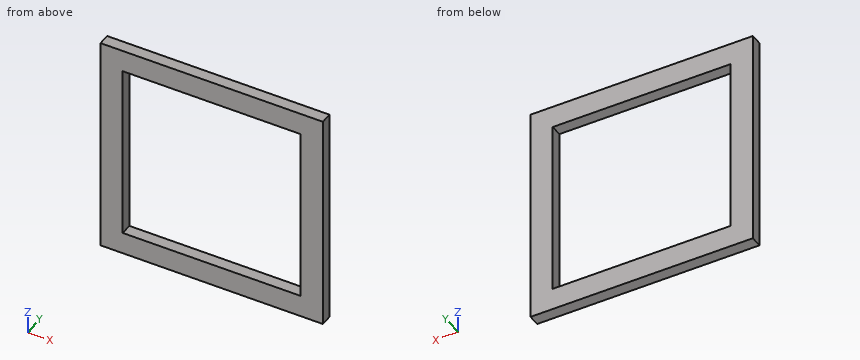
from build123d import *

# Parameters (mm, degrees)
SKETCH1_W           = 88.9
SKETCH1_H           = 88.9
SKETCH1_R           = 2.032
SKETCH1_W_2         = 63.5
SKETCH1_H_2         = 63.5
SKETCH1_W_3         = 50.8
SKETCH1_H_3         = 50.8
BOSS_EXTRUDE2_DEPTH = 3.175
BOSS_EXTRUDE3_START = 3.175
SKETCH1_4_W         = 63.5
SKETCH1_4_H         = 63.5
SKETCH1_4_W_2       = 50.8
SKETCH1_4_H_2       = 50.8
BOSS_EXTRUDE3_DEPTH = 3.302
SKETCH2_W           = 88.9
SKETCH2_H           = 88.9
CUT_EXTRUDE1_DEPTH  = 4.175


with BuildPart() as part:
    # Sketch1 → Boss-Extrude2 (new body)
    with BuildSketch(Plane(origin=(0, 0, 0), x_dir=(1, 0, 0), z_dir=(0, 1, 0))):
        Rectangle(SKETCH1_W, SKETCH1_H)
        with Locations((38.1, 38.1)):
            Circle(SKETCH1_R, mode=Mode.SUBTRACT)
        with Locations((-38.1, 38.1)):
            Circle(SKETCH1_R, mode=Mode.SUBTRACT)
        with Locations((38.1, -38.1)):
            Circle(SKETCH1_R, mode=Mode.SUBTRACT)
        with Locations((-38.1, -38.1)):
            Circle(SKETCH1_R, mode=Mode.SUBTRACT)
        Rectangle(SKETCH1_W_2, SKETCH1_H_2, mode=Mode.SUBTRACT)
        Rectangle(SKETCH1_W_3, SKETCH1_H_3)
        Rectangle(SKETCH1_W_2, SKETCH1_H_2)
        Rectangle(SKETCH1_W_3, SKETCH1_H_3, mode=Mode.SUBTRACT)
    extrude(amount=BOSS_EXTRUDE2_DEPTH)

    # Sketch1<4> → Boss-Extrude3 (add)
    with BuildSketch(Plane(origin=(0, 0, 0), x_dir=(1, 0, 0), z_dir=(0, 1, 0)).offset(BOSS_EXTRUDE3_START)):
        Rectangle(SKETCH1_4_W, SKETCH1_4_H)
        Rectangle(SKETCH1_4_W_2, SKETCH1_4_H_2, mode=Mode.SUBTRACT)
    extrude(amount=BOSS_EXTRUDE3_DEPTH)

    # Sketch2 → Cut-Extrude1 (cut, through all)
    with BuildSketch(Plane(origin=(0, 3.175, 0), x_dir=(1, 0, 0), z_dir=(0, 1, 0))):
        Rectangle(SKETCH2_W, SKETCH2_H)
    extrude(amount=-CUT_EXTRUDE1_DEPTH, mode=Mode.SUBTRACT)


solid = part.part
Work out the finished part from the listing and answer in its coordinate system (mm). Round coordinates to 2 decimals unless told otherwise and drop trailing zeros. Write each loop counter-clockwise with the first axis right and the second up, starting at its lowest first coordinate (ties: lowest second). Pieces come first, ordered by that corner, then holes. Notation, with made-up numbers: (-3.5, 32) - (4.5, 32) arc R10 ccw to (4.5, 46) - close; hole circle Ø8 at (-2.5, 2.5). An arc over 180 degrees is marked (long way). Answer in a Markdown table with one row per item. Add a question column.
1. Find the intervals of material crossed by line 1 along Z through (x, y) = (11, 5.35), in increasing order. Write a range as from..to.
2. A cutting plane is placed at A-A, the plane y = 3.85. Determine the outline of the cut face in (x, z).
3. Given pin 1 (5 mm diameter, centred on x = -3.5, z = -22.5, fed in from -Y), flat-ended and moving along its own axis, determine where the tip first touches the part or whether it passes through.
4. A cutting plane is placed at C-C, the plane z = -8. Determine the outline of the cut face in (x, y) (3 decimals), and give its area (3 significant figures).
5. A cutting plane is placed at B-B, the plane x = 16. Determine the outline of the cut face in (y, z) (3 decimals).
Worked out:
| question | item | result |
|---|---|---|
| 1 | line 1 | -31.75..-25.4, 25.4..31.75 |
| 2 | outline | (-31.75, -31.75) - (31.75, -31.75) - (31.75, 31.75) - (-31.75, 31.75) - close; hole (-25.4, -25.4) - (25.4, -25.4) - (25.4, 25.4) - (-25.4, 25.4) - close |
| 3 | pin 1 | through |
| 4 | outline | (-31.75, 3.175) - (-25.4, 3.175) - (-25.4, 6.477) - (-31.75, 6.477) - close; (25.4, 3.175) - (31.75, 3.175) - (31.75, 6.477) - (25.4, 6.477) - close |
| 4 | area | 41.9 mm^2 |
| 5 | outline | (3.175, -31.75) - (6.477, -31.75) - (6.477, -25.4) - (3.175, -25.4) - close; (3.175, 25.4) - (6.477, 25.4) - (6.477, 31.75) - (3.175, 31.75) - close |
